Verification items for the finished model (mm, model axes). A direction names the side the tool comes from. Round coordinates to 2 decimals unless told otherwise and drop trailing zeros. Write each loop counter-clockwise with the first axis right and the second up, starting at its lowest first coordinate (ties: lowest second). Pieces come first, ordered by that corner, then holes. Notation, with made-up numbers: M -17,32.25 L -7,32.25 A15 ccw -7,50.25 Z; hole C 37,42 d7. An arc over 180 degrees is marked long. One line per question, with ' | ' between items.
from build123d import *

# Parameters (mm, degrees)
F0_R     = 26.5
F1_DEPTH = 45
F2_ANGLE = 12.5
F4_DEPTH = 17.5
F6_DEPTH = 17.5
F7_R     = 5
F8_R     = 5


with BuildPart() as f1:
    # F0 (on Front) → F1 (new body)
    with BuildSketch(Plane.XZ):
        with BuildLine():
            ThreePointArc((-40.478678, -24.757054), (-28.191847, -26.283521), (-16.656806, -30.782313))
            ThreePointArc((-16.656806, -30.782313), (35, 0), (-16.656806, 30.782313))
            ThreePointArc((-16.656806, 30.782313), (-28.191847, 26.283521), (-40.478678, 24.757054))
            Line((-40.478678, 24.757054), (-475.64768, 24.987125))
            ThreePointArc((-475.64768, 24.987125), (-499.307017, 27.839125), (-521.619742, 36.20814))
            Line((-521.619742, 36.20814), (-609.903107, 81.976138))
            ThreePointArc((-609.903107, 81.976138), (-614.148891, 84.449185), (-618.13144, 87.327022))
            ThreePointArc((-618.13144, 87.327022), (-673.026094, 71.587801), (-640, 25))
            add(Edge.make_bspline(
                [(-640, -25), (-615, -30), (-545, 0), (-615, 30), (-640, 25)],
                knots=[0, 0, 0, 0, 65, 130, 130, 130, 130], degree=3))
            ThreePointArc((-640, -25), (-673.026094, -71.587801), (-618.13144, -87.327022))
            ThreePointArc((-618.13144, -87.327022), (-614.148891, -84.449185), (-609.903107, -81.976138))
            Line((-609.903107, -81.976138), (-521.619742, -36.20814))
            ThreePointArc((-521.619742, -36.20814), (-499.307017, -27.839125), (-475.64768, -24.987125))
            Line((-475.64768, -24.987125), (-40.478678, -24.757054))
        make_face()
        with Locations((-640, -60)):
            Circle(F0_R, mode=Mode.SUBTRACT)
        with Locations((-640, 60)):
            Circle(F0_R, mode=Mode.SUBTRACT)
        Circle(F0_R, mode=Mode.SUBTRACT)
    extrude(amount=F1_DEPTH)


with BuildPart() as f2_1:
    # F2: copy of F1
    add(f1.part.rotate(Axis((0, -45, 0), (0, -1, 0)), F2_ANGLE))


with BuildPart() as f4_tool:
    # F3 (on face) → F4 (new body)
    with BuildSketch(Plane.XZ.offset(45)):
        with BuildLine():
            Line((-41.5, -14.757592), (-41.5, 14.757592))
            Line((-41.5, 14.757592), (-502.440519, 15.001289))
            Line((-502.440519, 15.001289), (-592.404261, 61.640431))
            Line((-592.404261, 61.640431), (-606.211741, 35.00674))
            Line((-606.211741, 35.00674), (-564.373406, 13.316846))
            ThreePointArc((-564.373406, 13.316846), (-556.277146, 0), (-564.373406, -13.316846))
            Line((-564.373406, -13.316846), (-606.211741, -35.00674))
            Line((-606.211741, -35.00674), (-592.404261, -61.640431))
            Line((-592.404261, -61.640431), (-502.440519, -15.001289))
            Line((-502.440519, -15.001289), (-41.5, -14.757592))
        make_face()
    extrude(amount=-F4_DEPTH)


with BuildPart() as f1_1:
    add(f1.part)

    # F4: cut by f4_tool
    add(f4_tool.part, mode=Mode.SUBTRACT)


with BuildPart() as f2_1_1:
    add(f2_1.part)

    # F4: cut by f4_tool
    add(f4_tool.part, mode=Mode.SUBTRACT)


with BuildPart() as f6_tool:
    # F5 (on face) → F6 (new body)
    with BuildSketch(Plane(origin=(0, 0, 0), x_dir=(-1, 0, 0), z_dir=(0, 1, 0))):
        with BuildLine():
            Line((502.440519, 15.001289), (41.5, 14.757592))
            Line((41.5, 14.757592), (41.5, -14.757592))
            Line((41.5, -14.757592), (502.440519, -15.001289))
            Line((502.440519, -15.001289), (592.404261, -61.640431))
            Line((592.404261, -61.640431), (606.211741, -35.00674))
            Line((606.211741, -35.00674), (564.373406, -13.316846))
            ThreePointArc((564.373406, -13.316846), (556.277146, 0), (564.373406, 13.316846))
            Line((564.373406, 13.316846), (606.211741, 35.00674))
            Line((606.211741, 35.00674), (592.404261, 61.640431))
            Line((592.404261, 61.640431), (502.440519, 15.001289))
        make_face()
    extrude(amount=-F6_DEPTH)


with BuildPart() as f1_2:
    add(f1_1.part)

    # F6: cut by f6_tool
    add(f6_tool.part, mode=Mode.SUBTRACT)

    # F7
    f7_edges = [f1_2.edges().sort_by_distance(p)[0] for p in [
        (-271.970259, -17.5, 14.879441),
        (-41.5, -17.5, 0),
        (-271.970259, -17.5, -14.879441),
        (-547.42239, -17.5, 38.32086),
        (-547.42239, -17.5, -38.32086),
        (-599.308001, -17.5, -48.323585),
        (-585.292573, -17.5, -24.161793),
        (-599.308001, -17.5, 48.323585),
    ]]
    fillet(f7_edges, radius=F7_R)

    # F8
    f8_edges = [f1_2.edges().sort_by_distance(p)[0] for p in [
        (-599.308001, -27.5, -48.323585),
        (-547.42239, -27.5, -38.32086),
        (-271.970259, -27.5, -14.879441),
        (-585.292573, -27.5, 24.161793),
        (-599.308001, -27.5, 48.323585),
        (-547.42239, -27.5, 38.32086),
        (-271.970259, -27.5, 14.879441),
        (-41.5, -27.5, 0),
    ]]
    fillet(f8_edges, radius=F8_R)


with BuildPart() as f2_1_2:
    add(f2_1_1.part)

    # F6: cut by f6_tool
    add(f6_tool.part, mode=Mode.SUBTRACT)


solid = f1_2.part
1. Go/stop test with flat-tipped pins: P1, Ø6, axis at x = -502, y = -16, coming from the -Z side; P2, Ø3, axis at x = -285.5, z = 1, coming from the -Y side; P3, Ø6, axis at x = -421.5, y = -39, coming from the -Z side. Record where each tip stops, or that it passes through.
Results:
P1: stops at z = -29.41 | P2: stops at y = -27.5 | P3: stops at z = -24.96
2. Section check A-A, the plane x = 0. Record the cut outline in (y, z), then the cut area to 3 significant figures.
Results:
outline: M -45,-35 L 0,-35 L 0,-26.5 L -45,-26.5 Z; M -45,26.5 L 0,26.5 L 0,35 L -45,35 Z | area: 765 mm2
3. Thickness scan on line 1 (Z direction, x = -640, y = -25); line 2 (Z direction, x = -88, y = -32); line 3 (Z direction, x = 0, y = -23.5). Record the ranges inside material, lowest first.
Results:
line 1: z = -95 to -86.5, -33.5 to -25, 25 to 33.5, 86.5 to 95 | line 2: z = -24.78 to -14.76, 14.76 to 24.78 | line 3: z = -35 to -26.5, 26.5 to 35
4. Tool access check on faces 1 (the face through (-556.28, -6.16, -0.23)), 2 (the face through (-365, -27.5, 0)), 3 (the face through (-666.474, -22.185, 61.165)). Record the directions out of +Z, -Z, +X, -X, +Y, -Y that give a thin tool (end or side, any length) a straight path to the whole face; none if there is none.
Results:
face 1: +Y | face 2: -Y | face 3: +Y, -Y
5. Mould release check, pull along Z, two halves, no side actions. Record for faces 4 (the face through (-548.175, -29.004, 37.105)), 5 (the face through (-28.36, -22.18, -26.24)), 6 (the face through (-401, 0, -21)): pulls with the +Z half, pulls with the -Z half, needs draft (parallel to the pull), parting line crosses it, or undercut.
Results:
face 4: undercut | face 5: pulls with the -Z half | face 6: needs draft
